```python
from build123d import *

# Parameters (mm, degrees)
SKETCH1_R           = 1.5
SKETCH1_R_2         = 1.65
BOSS_EXTRUDE1_DEPTH = 3.175
FILLET1_R           = 10


with BuildPart() as part:
    # Sketch1 → Boss-Extrude1 (new body)
    with BuildSketch(Plane(origin=(0, 0, 0), x_dir=(1, 0, 0), z_dir=(0, 1, 0))):
        Polygon((-20, -190), (0, -190), (0, 0), (-129.696551146, 0), align=None)
        with Locations(Location((-65.10548978, -96.875, 0), (0, 0, 270))):
            Circle(SKETCH1_R, mode=Mode.SUBTRACT)
        with Locations(Location((-10, -175, 0), (0, 0, 270))):
            Circle(SKETCH1_R_2, mode=Mode.SUBTRACT)
        with Locations(Location((-35.10548978, -148.836524227, 0), (0, 0, 270))):
            Circle(SKETCH1_R, mode=Mode.SUBTRACT)
        with BuildLine():
            ThreePointArc((-10, -139.75), (-8.5, -141.25), (-10, -142.75))
            ThreePointArc((-10, -142.75), (-11.5, -141.25), (-10, -139.75))
        make_face(mode=Mode.SUBTRACT)
        with BuildLine():
            ThreePointArc((-10, -106), (-8.5, -107.5), (-10, -109))
            ThreePointArc((-10, -109), (-11.5, -107.5), (-10, -106))
        make_face(mode=Mode.SUBTRACT)
        with Locations(Location((-95.10548978, -44.913475773, 0), (0, 0, 270))):
            Circle(SKETCH1_R, mode=Mode.SUBTRACT)
        with Locations(Location((-116.706170089, -7.5, 0), (0, 0, 270))):
            Circle(SKETCH1_R, mode=Mode.SUBTRACT)
        with Locations(Location((-68.353085045, -7.5, 0), (0, 0, 270))):
            Circle(SKETCH1_R, mode=Mode.SUBTRACT)
        Polygon((-20, -15), (-20, -160), (-103.715789032, -15), align=None, mode=Mode.SUBTRACT)
        with BuildLine():
            ThreePointArc((-10, -72.25), (-8.5, -73.75), (-10, -75.25))
            ThreePointArc((-10, -75.25), (-11.5, -73.75), (-10, -72.25))
        make_face(mode=Mode.SUBTRACT)
        with Locations(Location((-10, -40, 0), (0, 0, 270))):
            Circle(SKETCH1_R_2, mode=Mode.SUBTRACT)
        with Locations(Location((-30, -7.5, 0), (0, 0, 270))):
            Circle(SKETCH1_R, mode=Mode.SUBTRACT)
        with Locations(Location((-10, -7.5, 0), (0, 0, 270))):
            Circle(SKETCH1_R, mode=Mode.SUBTRACT)
    extrude(amount=BOSS_EXTRUDE1_DEPTH)

    # Fillet1
    fillet1_edges = [part.edges().sort_by_distance(p)[0] for p in [
        (-20, 1.5875, 15),
        (-103.715789032, 1.5875, 15),
        (-20, 1.5875, 160),
        (-129.696551146, 1.5875, 0),
        (0, 1.5875, 0),
        (0, 1.5875, 190),
        (-20, 1.5875, 190),
    ]]
    fillet(fillet1_edges, radius=FILLET1_R)


solid = part.part
```
CAD build for the part. Positions are in the model's coordinates, mm. A direction names the side the tool comes from. Give positions to 0.01 mm unless a question says otherwise; leave off trailing zeros. Order: outer loops, then holes, each group sorted by start corner. A loop starts at its lowest first (then second) coordinate and runs counter-clockwise, first axis right, second up.
(1) Saw through at B-B, the plane x = -72.5. Give the cut face in (y, z) (3 decimals), then the cut area to 3 significant figures.
(2) Flat gauge pins, fed straight in: pin 1 (4 mm diameter, centred on x = -10, z = 40, fed in from +Y) (3 decimals); pin 2 (1 mm diameter, centred on y = 1.5, z = 100.5, fed in from -X); pin 3 (1 mm diameter, centred on x = -55.5, y = 1.5, fed in from +Z). Where does each tip first touch, or does it go through?
(3) Saw through at D-D, the plane x = -105. Give the cut face in (y, z) (3 decimals).
(4) Tool access for faces 1 (the cylindrical face through (-94.98, 1.61, 19.87)), 2 (the flat face through (-72.65, 1.57, 98.81)): list every direction of +Z, -Z, +X, -X, +Y, -Y with a clear straight run to the whole face (end or side of a thin tool).
(5) Saw through at C-C, the plane y = 2.5. State how many separate pieces and enclosed holes the cut face has, then the cut area to 3 significant figures.
(6) Drill centre lines: L1, parallel to X at y = 1.3, z = 40; L2, parallel to X at y = 0.15, z = 108.5; L3, parallel to X at y = 2.15, z = 7.5. Where is each one in solid material? Low to high.
(7) Saw through at A-A, the plane z = 48.5. Give the cut face in (x, y) (3 decimals), then the cut area to 3 significant figures.
(8) Mould opens along X. For faces 3 (the flat face through (-66.463, 1.565, 79.524)), 4 (the cylindrical face through (-121.11, 1.61, 5.13)), 5 (the cylindrical face through (-27.589, 1.61, 132.385)), 6 (the flat face through (-61, 0, 95)) say: released by +X, released by -X, zero draft, split by the parting line, or undercut.
Results found:
1. outline: (0, 0) - (3.175, 0) - (3.175, 15) - (0, 15) - close; (0, 69.067) - (3.175, 69.067) - (3.175, 99.067) - (0, 99.067) - close
1. area: 143 mm2
2. pin 1: stops at y = 3.175
2. pin 2: stops at x = -71.96
2. pin 3: stops at z = 129.38
3. outline: (0, 0) - (3.175, 0) - (3.175, 42.776) - (0, 42.776) - close
4. face 1: +Y, -Y
4. face 2: +Z, -X, +Y, -Y
5. separate pieces: 1
5. enclosed holes: 13
5. area: 8,280 mm2
6. L1: x = -106.6 to -89.28, -20 to -11.65, -8.35 to 0
6. L2: x = -67.05 to -49.73, -20 to -11.12, -8.88 to 0
6. L3: x = -122.06 to -118.21, -115.21 to -69.85, -66.85 to -31.5, -28.5 to -11.5, -8.5 to -0.32
7. outline: (-101.695, 0) - (-84.375, 0) - (-84.375, 3.175) - (-101.695, 3.175) - close; (-20, 0) - (0, 0) - (0, 3.175) - (-20, 3.175) - close
7. area: 118 mm2
8. face 3: undercut
8. face 4: released by -X
8. face 5: undercut
8. face 6: zero draft
